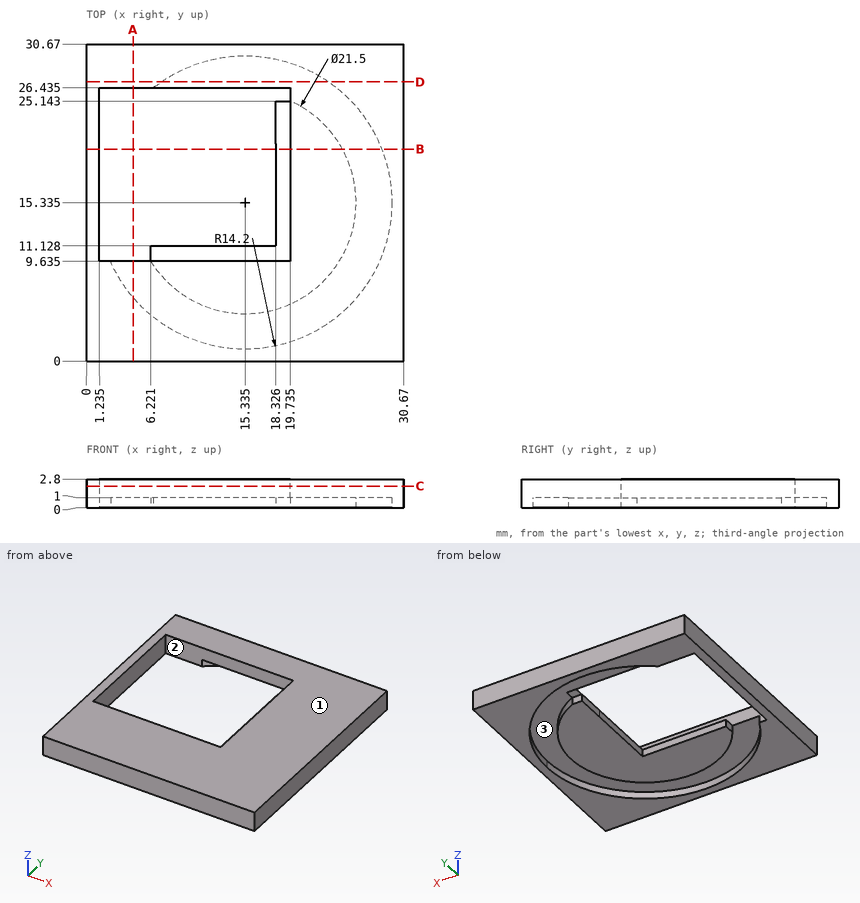
Source: three-view drawing plus pictorial views. Frame: mm from the lowest corner of the part. Coordinates: 2 decimals unless noted, no trailing zeros. Order: outer loops, then holes, each group sorted by start corner. A loop starts at its lowest first (then second) coordinate and runs counter-clockwise, first axis right, second up.
Item 1: Pull-direction query (X, two-part tool) for the marked faces 1, 2 and 3; classes: pulls with the +X half, pulls with the -X half, needs draft (parallel to the pull), parting line crosses it, or undercut.
Output values:
face 1: needs draft
face 2: undercut
face 3: undercut
Item 2: Cut plane D-D (y = 27). Return loops of the section in (x, z).
Output values:
outline: (0, 0) - (7.24, 0) - (7.24, 1) - (23.43, 1) - (23.43, 0) - (30.67, 0) - (30.67, 2.8) - (0, 2.8) - close
Item 3: Material intervals for line 1 (Y direction, x = 7, z = 2.3) (1 decimal); line 2 (X direction, y = 23, z = 1.9) (1 decimal); line 3 (Y direction, x = 14, z = 0.5), sorted ascending.
Output values:
line 1: y = 0 to 9.6, 26.4 to 30.7
line 2: x = 0 to 1.2, 19.7 to 30.7
line 3: y = 0 to 1.2, 4.67 to 11.13, 29.47 to 30.67
Item 4: Cut plane C-C (z = 2.1). Return loops of the section in (x, y) (1 decimal).
Output values:
outline: (0, 0) - (30.7, 0) - (30.7, 30.7) - (0, 30.7) - close; hole (1.2, 9.6) - (19.7, 9.6) - (19.7, 26.4) - (1.2, 26.4) - close
Item 5: Cut plane A-A (x = 4.5). Return loops of the section in (y, z) (1 decimal).
Output values:
outline: (0, 0) - (6.2, 0) - (6.2, 1) - (9.6, 1) - (9.6, 2.8) - (0, 2.8) - close; (26.4, 0) - (30.7, 0) - (30.7, 2.8) - (26.4, 2.8) - close
Item 6: Cut plane B-B (y = 20.5). Return loops of the section in (x, z) (1 decimal).
Output values:
outline: (0, 0) - (1.2, 0) - (1.2, 2.8) - (0, 2.8) - close; (18.3, 0) - (24.8, 0) - (24.8, 1) - (28.6, 1) - (28.6, 0) - (30.7, 0) - (30.7, 2.8) - (19.7, 2.8) - (19.7, 1) - (18.3, 1) - close
